```python
from build123d import *

# Parameters (mm, degrees)
SCHIZZO1_R                   = 5.5
ESTRUSIONE_ESTRUSIONE1_DEPTH = 30
SCHIZZO2_R                   = 4
TAGLIO_ESTRUSIONE1_DEPTH     = 31
SMUSSO1_SIZE                 = 0.5


with BuildPart() as part:
    # Schizzo1 → Estrusione-Estrusione1 (new body)
    with BuildSketch(Plane.XY):
        Circle(SCHIZZO1_R)
    extrude(amount=ESTRUSIONE_ESTRUSIONE1_DEPTH)

    # Schizzo2 → Taglio-Estrusione1 (cut, through all)
    with BuildSketch(Plane.XY.offset(30)):
        Circle(SCHIZZO2_R)
    extrude(amount=-TAGLIO_ESTRUSIONE1_DEPTH, mode=Mode.SUBTRACT)

    # Smusso1
    smusso1_edges = [part.edges().sort_by_distance(p)[0] for p in [
        (-5.5, 0, 0),
        (-5.5, 0, 30),
    ]]
    chamfer(smusso1_edges, length=SMUSSO1_SIZE)


solid = part.part
```
Geometry: final body of the model. Coordinates: model frame, mm. Round coordinates to 2 decimals unless told otherwise and drop trailing zeros. Loops run counter-clockwise (first coordinate to the right, second up) from the corner with the lowest first, then second, coordinate; pieces in that order, holes last. Notation, with made-up numbers: (48, 34.25) -> (72, 34.25) arc R13 cw to (72, 39.25) -> close; hole circle Ø9 at (-33, 58). An arc over 180 degrees is marked (long way). Use one line per item in the form item = value.
Item 1: Contact query for flat-ended pins moving along their axis: pin 1 Ø2 at (x, z) = (-2.5, 14.5) entering from +Y; pin 2 Ø5 at (x, z) = (4.5, 20) entering from +Y. Output: stop coordinate, or through.
Evaluation:
pin_1 = 5.29
pin_2 = 5.12
Item 2: Draft query along X for faces 1 (the cylindrical face through (-1.19, -5.37, 14.8)), 2 (the cylindrical face through (-0.867, -3.905, 15.21)). Return one class per face: released by +X, released by -X, zero draft, split by the parting line, or undercut.
Evaluation:
face_1 = split by the parting line
face_2 = undercut
Item 3: Cut plane A-A on y = 0. Output: boundary loops of the cut face in (x, z), then the cut area to 3 significant figures.
Evaluation:
outline = (-5.5, 0.5) -> (-5, 0) -> (-4, 0) -> (-4, 30) -> (-5, 30) -> (-5.5, 29.5) -> close; (4, 0) -> (5, 0) -> (5.5, 0.5) -> (5.5, 29.5) -> (5, 30) -> (4, 30) -> close
area = 89.5 mm2
Item 4: Cut plane C-C on z = 7.5. Output: boundary loops of the cut face in (x, y), then the cut area to 3 significant figures.
Evaluation:
outline = circle Ø11 at (0, 0); hole circle Ø8 at (0, 0)
area = 44.8 mm2
Item 5: Material intervals for probe 1 along Y at (x, z) = (0, 10.5); probe 2 along Y at (x, z) = (0.75, 14.25); probe 3 along X at (y, z) = (-2.5, 4), sorted ascending.
Evaluation:
probe_1 = -5.5 to -4, 4 to 5.5
probe_2 = -5.45 to -3.93, 3.93 to 5.45
probe_3 = -4.9 to -3.12, 3.12 to 4.9
